Verification items for this drawing (mm, ordinates from the low corner). A direction names the side the tool comes from. Give positions to 0.01 mm unless a question says otherwise; leave off trailing zeros. Loops run counter-clockwise (first coordinate to the right, second up) from the corner with the lowest first, then second, coordinate; pieces in that order, holes last. Notation, with made-up numbers: (-6, 32.5) -> (41, 32.5) arc R19 cw to (41, 43.5) -> close; hole circle Ø10 at (71.25, -14.75). An arc over 180 degrees is marked (long way). Use one line per item in the form item = value. Start each with the question number.
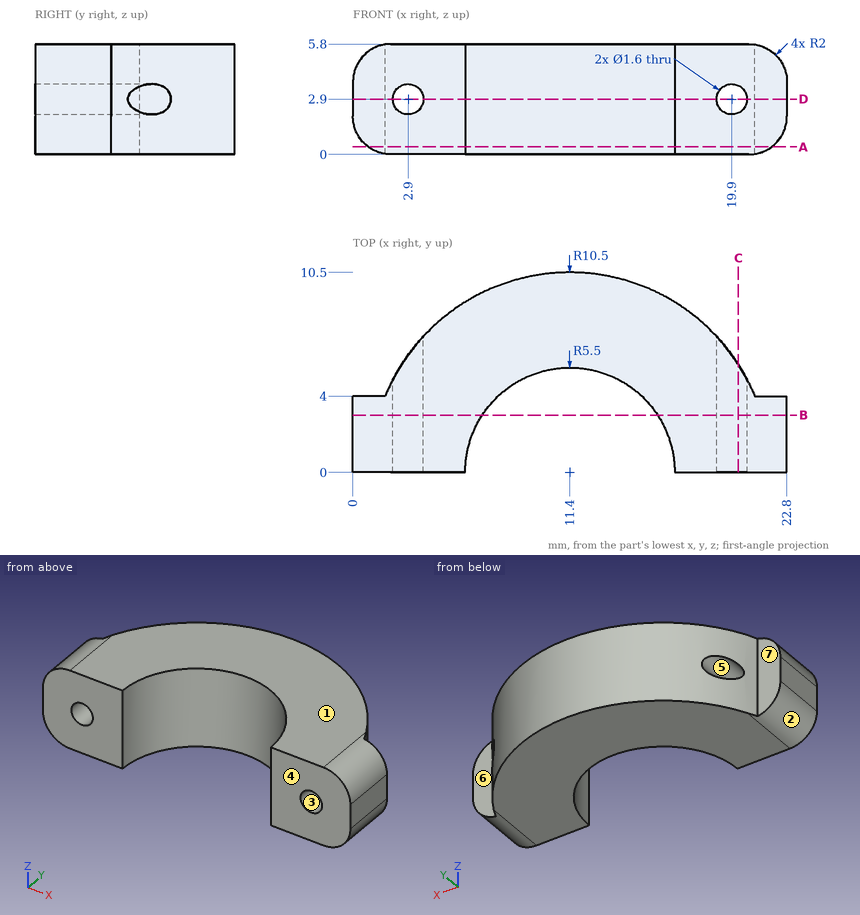
Item 1: Material ranges on line 1 (Z direction, x = 19.9, y = 5.25); line 2 (X direction, y = 2.75, z = 2.7); line 3 (X direction, y = 5, z = 0.4), recorded low to high.
Item 2: Sectioned sample at B-B, the plane y = 3. Enter the section's corners in (x, z), and give its area (3 significant figures).
Item 3: Sectioned sample at A-A, the plane z = 0.4. Enter the section's corners in (x, y), and give its area (3 significant figures).
Item 4: Tool access check on the marked faces 5, 6 and 7. Record the directions out of +Z, -Z, +X, -X, +Y, -Y that give a thin tool (end or side, any length) a straight path to the whole face; none if there is none.
Item 5: Sectioned sample at C-C, the plane x = 20.25. Enter the section's corners in (y, z), and give its area (3 significant figures).
Item 6: Gauge pin test, flat ends, axial feed: pin 1 Ø1 at (y, z) = (8.5, 3) entering from -X; pin 2 Ø1 at (x, z) = (19.9, 2.9) entering from +Y; pin 3 Ø0.5 at (x, z) = (22, 2) entering from +Y; pin 4 Ø3 at (x, z) = (20.5, 0.5) entering from +Y (3 decimals). Record the tip position at first contact, or that the pin passes through.
Item 7: Draft check along Z on the marked faces 1, 2, 3 and 4. Enter one of: +Z half, -Z half, draft (parallel to the pull), parting line (faces both ways), or undercut.
Item 8: Sectioned sample at D-D, the plane z = 2.9. Enter the section's corners in (x, y).
Outcome:
q1.line_1 = 0 to 2.1, 3.7 to 5.8
q1.line_2 = 0 to 2.13, 3.67 to 6.64, 16.16 to 19.13, 20.67 to 22.8
q1.line_3 = 2.17 to 9.11, 13.69 to 20.63
q2.outline = (0, 2) arc R2 ccw to (2, 0) -> (6.79, 0) -> (6.79, 5.8) -> (2, 5.8) arc R2 ccw to (0, 3.8) -> close; (16.01, 0) -> (20.8, 0) arc R2 ccw to (22.8, 2) -> (22.8, 3.8) arc R2 ccw to (20.8, 5.8) -> (16.01, 5.8) -> close; hole circle Ø1.6 at (2.9, 2.9); hole circle Ø1.6 at (19.9, 2.9)
q2.area = 71.3 mm^2
q3.outline = (0.8, 0) -> (5.9, 0) arc R5.5 cw to (16.9, 0) -> (22, 0) -> (22, 4) -> (21.11, 4) arc R10.5 ccw to (1.69, 4) -> (0.8, 4) -> close
q3.area = 129 mm^2
q4.face_5 = +Y, -Y
q4.face_6 = +Z, -Z, +X, +Y
q4.face_7 = +Z, -Z, -X, +Y
q5.outline = (0, 0) -> (5.65, 0) -> (5.65, 2.18) -> (0, 2.18) -> close; (0, 3.62) -> (5.65, 3.62) -> (5.65, 5.8) -> (0, 5.8) -> close
q5.area = 24.6 mm^2
q6.pin_1 = 4.6
q6.pin_2 = through
q6.pin_3 = 4
q6.pin_4 = 7.245
q7.face_1 = +Z half
q7.face_2 = -Z half
q7.face_3 = undercut
q7.face_4 = draft
q8.outline = (0, 0) -> (2.1, 0) -> (2.1, 4.87) arc R10.5 ccw to (1.69, 4) -> (0, 4) -> close; (3.7, 0) -> (5.9, 0) arc R5.5 cw to (16.9, 0) -> (19.1, 0) -> (19.1, 7.14) arc R10.5 ccw to (3.7, 7.14) -> close; (20.7, 0) -> (22.8, 0) -> (22.8, 4) -> (21.11, 4) arc R10.5 ccw to (20.7, 4.87) -> close
